Print and shaded views of the part. All mm, measured from the part's lowest x, y and z. A direction names the side the tool comes from. Coordinates: 2 decimals unless noted, no trailing zeros. Loops run counter-clockwise (first coordinate to the right, second up) from the corner with the lowest first, then second, coordinate; pieces in that order, holes last.
1) Saw through at A-A, the plane y = 22.5. Write the cut outline in (x, z).
2) Saw through at B-B, the plane z = 254.06. Write the cut outline in (x, y), and give its area (3 significant figures).
3) Wall check: line 1 along Y through (x, z) = (1, 254); line 2 along X through (y, z) = (12, 182). Give the ranges that are in metal, low to high.
4) Pin check, flat tip, straight feed: pin 1 Ø3.5 at (y, z) = (9, 254.06) entering from -X (1 decimal). Stop position of the tip, or through.
5) Which spindle directions (+Z, -Z, +X, -X, +Y, -Y) get a long thin tool onto all of the face, cutting with end or side? Do the marked faces 1 and 2. Say none if no direction does.
6) Saw through at D-D, the plane z = 106.5. Write the cut outline in (x, y).
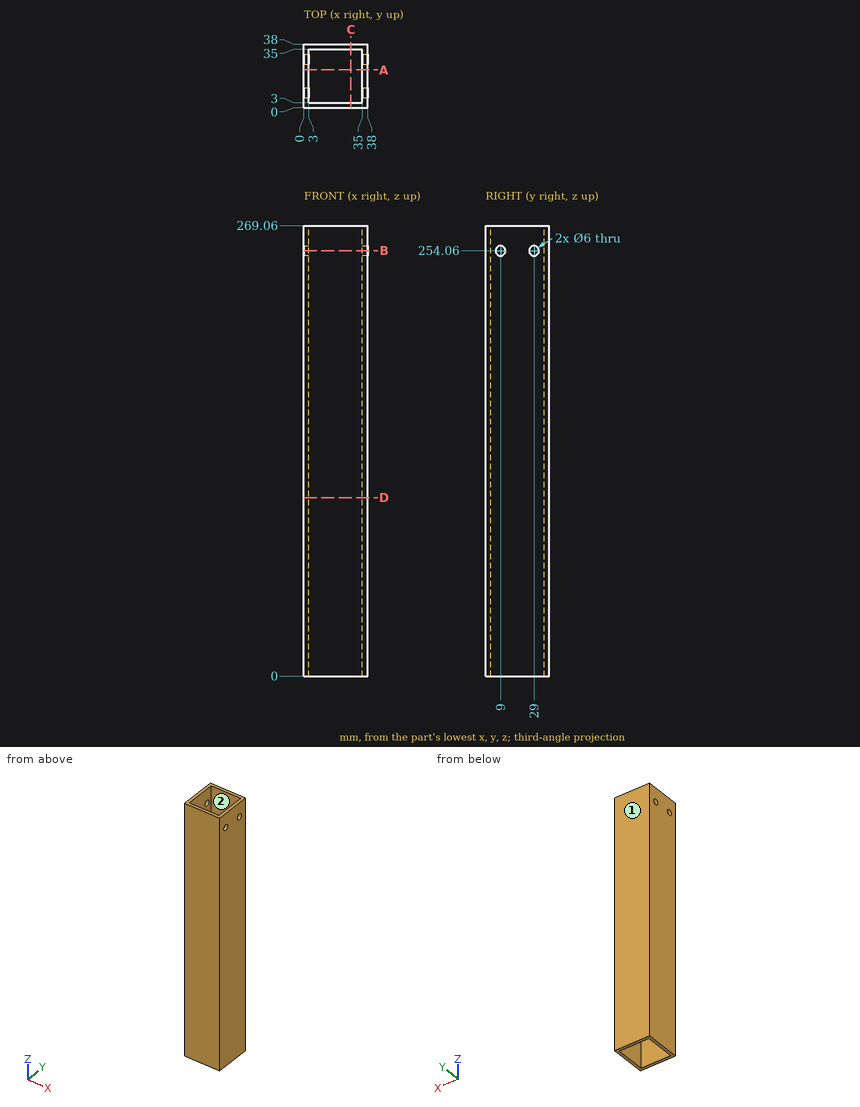
Data:
1. outline: (0, 0) - (3, 0) - (3, 269.06) - (0, 269.06) - close; (35, 0) - (38, 0) - (38, 269.06) - (35, 269.06) - close
2. outline: (0, 0) - (38, 0) - (38, 6) - (35, 6) - (35, 3) - (3, 3) - (3, 6) - (0, 6) - close; (0, 12) - (3, 12) - (3, 26) - (0, 26) - close; (0, 32) - (3, 32) - (3, 35) - (35, 35) - (35, 32) - (38, 32) - (38, 38) - (0, 38) - close; (35, 12) - (38, 12) - (38, 26) - (35, 26) - close
2. area: 348 mm2
3. line 1: y = 0 to 6, 12 to 26, 32 to 38
3. line 2: x = 0 to 3, 35 to 38
4. pin 1: passes through
5. face 1: +Z, -Z, +X, -X, +Y
5. face 2: +Z, -Z
6. outline: (0, 0) - (38, 0) - (38, 38) - (0, 38) - close; hole (3, 3) - (35, 3) - (35, 35) - (3, 35) - close
